The listing builds one solid part. Answer for the finished solid, in the listing's coordinates (mm). Face numbers are marked on the shaded views. Round coordinates to 2 decimals unless told otherwise and drop trailing zeros. Write each loop counter-clockwise with the first axis right and the second up, starting at its lowest first coordinate (ties: lowest second). Pieces come first, ordered by that corner, then holes. Notation, with made-up numbers: M -16.5,-29.5 L 41.5,-29.5 A34 cw 41.5,4.5 Z; hole C 72.25,69 d1. An arc over 180 degrees is marked long. Write each question's results on one line, items separated by ' | '.
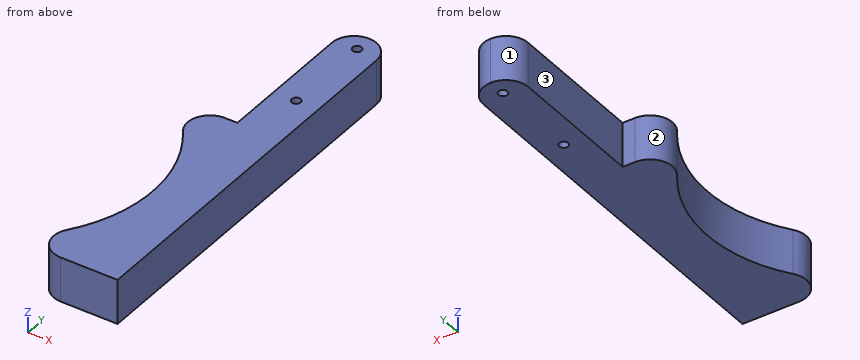
from build123d import *

# Parameters (mm, degrees)
ESQUISSE1_W             = 10
ESQUISSE1_H             = 90
BOSS_EXTRU_1_DEPTH      = 10
ESQUISSE2_R             = 1
ENL_V_MAT_EXTRU_1_DEPTH = 10
CONG_1_R                = 5
BOSS_EXTRU_2_DEPTH      = 10
CONG_2_R                = 5


with BuildPart() as part:
    # Esquisse1 → Boss.-Extru.1 (new body)
    with BuildSketch(Plane.XY):
        with Locations((5, 45)):
            Rectangle(ESQUISSE1_W, ESQUISSE1_H)
    extrude(amount=BOSS_EXTRU_1_DEPTH)

    # Esquisse2 → Enlèv. mat.-Extru.1 (cut)
    with BuildSketch(Plane.XY.offset(10)):
        with Locations((5, 66)):
            Circle(ESQUISSE2_R)
        with Locations((5, 86)):
            Circle(ESQUISSE2_R)
    extrude(amount=-ENL_V_MAT_EXTRU_1_DEPTH, mode=Mode.SUBTRACT)

    # Congé1
    cong_1_edges = [part.edges().sort_by_distance(p)[0] for p in [
        (10, 90, 5),
        (0, 90, 5),
    ]]
    fillet(cong_1_edges, radius=CONG_1_R - 0.0001)  # a hair under: the kernel refuses the full size

    # Esquisse3 → Boss.-Extru.2 (add)
    with BuildSketch(Plane.XY.offset(10)):
        with BuildLine():
            Line((0, 0), (0, 54))
            Line((0, 54), (-15, 54))
            ThreePointArc((-15, 54), (-0.590052515, 27), (-15, 0))
            Line((-15, 0), (0, 0))
        make_face()
    extrude(amount=-BOSS_EXTRU_2_DEPTH)

    # Congé2
    cong_2_edges = [part.edges().sort_by_distance(p)[0] for p in [
        (-15, 0, 5),
        (-15, 54, 5),
    ]]
    fillet(cong_2_edges, radius=CONG_2_R)


solid = part.part
1) Section C-C (x = -5) is taken. Determine the outline of the cut face in (y, z).
Return value:
outline: M 0.55,0 L 10.65,0 L 10.65,10 L 0.55,10 Z; M 43.35,0 L 53.45,0 L 53.45,10 L 43.35,10 Z
2) Each of these flat-tipped pins is pushed along its axis until it touches: pin 1 (3 mm diameter, centred on x = 4, y = 11.5, fed in from -Z); pin 2 (4 mm diameter, centred on y = 39.5, z = 3.5, fed in from -X); pin 3 (1.5 mm diameter, centred on y = 26.5, z = 8, fed in from -X); pin 4 (5 mm diameter, centred on y = 77, z = 4.5, fed in from -X). Where does it stop, or does it pass through?
Return value:
pin 1: z = 0 | pin 2: x = -4 | pin 3: x = -0.61 | pin 4: x = 0
3) Section D-D (y = 42) is taken. Determine the outline of the cut face in (x, z).
Return value:
outline: M -4.26,0 L 10,0 L 10,10 L -4.26,10 Z
4) Find the intervals of material crossed by line 1 (Y direction, x = 5, z = 5.25); line 2 (X direction, y = 66, z = 6.25); line 3 (Y direction, x = 4.5, z = 8), in increasing order.
Return value:
line 1: 0 to 65, 67 to 85, 87 to 90 | line 2: 0 to 4, 6 to 10 | line 3: 0 to 65.13, 66.87 to 85.13, 86.87 to 89.97
5) Section A-A (y = 66) is taken. Determine the outline of the cut face in (x, z), then the cut area to 3 significant figures.
Return value:
outline: M 0,0 L 4,0 L 4,10 L 0,10 Z; M 6,0 L 10,0 L 10,10 L 6,10 Z | area: 80.0 mm²
6) The mould has two halves that part along Y. Classify the marked faces 1, 2 and 3: +Y half, -Y half, draft (parallel to the pull), parting line (faces both ways), or undercut.
Return value:
face 1: +Y half | face 2: undercut | face 3: draft
7) Section B-B (z = 4.75) is taken. State how many separate pieces and enclosed holes the cut face has, then the cut area to 3 significant figures.
Return value:
separate pieces: 1 | enclosed holes: 2 | area: 1,090 mm²
